The model under review builds one solid part; all positions refer to its coordinate system, in mm. A direction names the side the tool comes from. Round coordinates to 2 decimals unless told otherwise and drop trailing zeros. Write each loop counter-clockwise with the first axis right and the second up, starting at its lowest first coordinate (ties: lowest second). Pieces come first, ordered by that corner, then holes. Notation, with made-up numbers: (-17.75, -10) -> (-7.75, -10) arc R12 cw to (-7.75, 12) -> close; hole circle Ø5 at (-32, 19.25). An arc over 180 degrees is marked (long way). Answer as a JSON object with one key per item and string values. Group by question number.
1) Mouldability with a two-part tool opening along Z and no side actions: class faces 4 (the flat face through (54.74, -34.51, 24.15)), 5 (the cylindrical face through (49.4, -8.57, 2.46)), 6 (the cylindrical face through (34.83, -8.6, 57.29)) as pulls with the +Z half, pulls with the -Z half, needs draft (parallel to the pull), parting line crosses it, or undercut.
2) We need section B-B, the plane z = 46. Write out the cut boundary in (x, y), then the cut area to 3 significant figures.
3) Machinability: for faces 1 (the cylindrical face through (9.977, -8.57, 16.697)), 2 (the cylindrical face through (49.4, -61.43, 2.46)), 3 (the flat face through (33.433, -34.51, 63.771)), which of the approach directions +Z, -Z, +X, -X, +Y, -Y give a long, thin tool a straight path to every point of the face, cutting with its end or side? Answer none if there is none.
4) Insertion check: pin 1 Ø6 at (x, z) = (25, 48) entering from +Y; pin 2 Ø10 at (x, z) = (33.5, 39) entering from +Y; pin 3 Ø1.1 at (y, z) = (-47, 2.5) entering from +X; pin 4 Ø4 at (x, y) = (65.5, -25.5) entering from -Z. Each pin has a flat end and moves straight along its axis. Give the tip position at first contact, or say it passes through.
5) We need section A-A, the plane y = -37. Count the separate pieces of the cut face and the enclosed holes in it, then the cut area to 3 significant figures.
6) To check wall thickness, follow probe 1 along Y at (x, z) = (24, 49); probe 2 along Z at (x, y) = (17, -42); probe 3 along Z at (x, y) = (53, -14.5). State the ranges of each line that lie inside material, in increasing order. Write a range as [from, to].
from build123d import *

# Parameters (mm, degrees)
PAD_DEPTH       = 70
POCKET_DEPTH    = 28.2506186199
FILLET_R        = 2
FILLET001_R     = 1
FILLET002_R     = 2
FILLET003_R     = 2
SKETCH002_W     = 34.4087464699
SKETCH002_H     = 54
POCKET001_DEPTH = 5
SKETCH003_W     = 39.3291895531
SKETCH003_H     = 54
POCKET002_DEPTH = 5
SKETCH004_W     = 31.3073233784
SKETCH004_H     = 54
POCKET003_DEPTH = 5
FILLET004_R     = 2
FILLET005_R     = 2


with BuildPart() as part:
    # Sketch → Pad (new body)
    with BuildSketch(Plane.XZ):
        Polygon((0, 0), (30, 68.7386354243), (61.2704610896, 23.4931023493), (71.9648598164, 30.8843022432), (71.9648598164, 35.8843022432), (76.9648598164, 35.8843022432), (76.9648598164, 28.2619948796), (60, 16.5371028798), (30.9913221648, 58.5100398536), (7.6376261583, 5), (60, 5), (60, 0), align=None)
    extrude(amount=PAD_DEPTH)

    # Sketch001 (on Face3 of Pad) → Pocket (cut, through all)
    with BuildSketch(Plane(origin=(8.8177286613, 0, -12.7584570195), x_dir=(-0.8226460559, 0, -0.568553838), z_dir=(-0.568553838, 0, 0.8226460559))):
        Polygon((-90.2609966662, 57.5), (-65.2609966662, 44), (-65.2609966662, 26), (-90.2609966662, 12.5), align=None)
    extrude(amount=-POCKET_DEPTH, mode=Mode.SUBTRACT)

    # Fillet
    fillet_edges = [part.edges().sort_by_distance(p)[0] for p in [
        (60, -35, 5),
        (60, -35, 0),
        (30, -35, 68.738635),
        (0, -35, 0),
        (60, -35, 16.537103),
        (71.96486, -35, 35.884302),
        (76.96486, -60.813023, 28.261995),
        (76.96486, -9.186977, 28.261995),
    ]]
    fillet(fillet_edges, radius=FILLET_R)

    # Fillet001
    fillet001_edges = [part.edges().sort_by_distance(p)[0] for p in [
        (61.270461, -35, 23.493102),
        (76.96486, -35, 35.884302),
        (76.96486, -35, 34.339943),
        (71.96486, -35, 30.884302),
    ]]
    fillet(fillet001_edges, radius=FILLET001_R)

    # Fillet002
    fillet002_edges = [part.edges().sort_by_distance(p)[0] for p in [
        (7.637626, -35, 5),
    ]]
    fillet(fillet002_edges, radius=FILLET002_R)

    # Fillet003
    fillet003_edges = [part.edges().sort_by_distance(p)[0] for p in [
        (65.347199, -35, 20.232703),
    ]]
    fillet(fillet003_edges, radius=FILLET003_R)

    # Sketch002 (on Face29 of Fillet003) → Pocket001 (cut)
    with BuildSketch(Plane(origin=(52.4527324283, 0, 36.2515593688), x_dir=(-0.568553838, 0, 0.8226460559), z_dir=(0.8226460559, 0, 0.568553838))):
        with Locations((10.6953254156, 35)):
            Rectangle(SKETCH002_W, SKETCH002_H)
    extrude(amount=-POCKET001_DEPTH, mode=Mode.SUBTRACT)

    # Sketch003 (on Face20 of Pocket001) → Pocket002 (cut)
    with BuildSketch(Plane(origin=(4.582575695, 0, -2), x_dir=(0.4, 0, 0.916515139), z_dir=(0.916515139, 0, -0.4))):
        with Locations((38.3572713981, 35)):
            Rectangle(SKETCH003_W, SKETCH003_H)
    extrude(amount=-POCKET002_DEPTH, mode=Mode.SUBTRACT)

    # Sketch004 (on Face17 of Pocket002) → Pocket003 (cut)
    with BuildSketch(Plane(origin=(0, 0, 5), x_dir=(-1, 0, 0), z_dir=(0, 0, 1))):
        with Locations((-34.3463383108, 35)):
            Rectangle(SKETCH004_W, SKETCH004_H)
    extrude(amount=-POCKET003_DEPTH, mode=Mode.SUBTRACT)

    # Fillet004
    fillet004_edges = [part.edges().sort_by_distance(p)[0] for p in [
        (54.096861, -8, 29.475532),
        (34.533637, -8, 57.781752),
        (34.533637, -62, 57.781752),
        (54.096861, -62, 29.475532),
        (18.692677, -62, 2.5),
        (18.692677, -8, 2.5),
        (50, -8, 2.5),
        (50, -62, 2.5),
        (9.768358, -62, 16.132121),
        (9.768358, -8, 16.132121),
        (25.500034, -8, 52.177919),
        (25.500034, -62, 52.177919),
    ]]
    fillet(fillet004_edges, radius=FILLET004_R)

    # Fillet005
    fillet005_edges = [part.edges().sort_by_distance(p)[0] for p in [
        (30.991322, -35, 58.51004),
    ]]
    fillet(fillet005_edges, radius=FILLET005_R)


solid = part.part
Here are the results:
{
 "1": {"face 4": "undercut", "face 5": "needs draft", "face 6": "pulls with the -Z half"},
 "2": {"outline": "(20.08, -70) -> (25.53, -70) -> (25.53, -62) -> (20.08, -62) -> close; (20.08, -8) -> (25.53, -8) -> (25.53, 0) -> (20.08, 0) -> close; (39.64, -70) -> (45.72, -70) -> (45.72, -62) -> (39.64, -62) -> close; (39.64, -8) -> (45.72, -8) -> (45.72, 0) -> (39.64, 0) -> close", "area": "185 mm^2"},
 "3": {"face 1": "+Z", "face 2": "+Z, -Z", "face 3": "+Z, +Y, -Y"},
 "4": {"pin 1": "stops at y = 0", "pin 2": "passes through", "pin 3": "stops at x = 60", "pin 4": "stops at z = 18.96"},
 "5": {"separate pieces": "5", "enclosed holes": "0", "area": "385 mm^2"},
 "6": {"probe 1": "y = [-70, -62], [-8, 0]", "probe 2": "z = [0, 5]", "probe 3": "z = [0, 5], [26.67, 28.72]"}
}
